from build123d import *

# Parameters (mm, degrees)
SZKIC1_R                    = 15
DODANIE_WYCI_GNI_CIE1_DEPTH = 33
SZKIC2_R                    = 20
DODANIE_WYCI_GNI_CIE2_DEPTH = 2
SZKIC3_R                    = 44
DODANIE_WYCI_GNI_CIE3_DEPTH = 15
SZKIC4_R                    = 15
DODANIE_WYCI_GNI_CIE4_DEPTH = 10


with BuildPart() as part:
    # Szkic1 → Dodanie-wyciągnięcie1 (new body)
    with BuildSketch(Plane.XY):
        Circle(SZKIC1_R)
    extrude(amount=DODANIE_WYCI_GNI_CIE1_DEPTH)

    # Szkic2 → Dodanie-wyciągnięcie2 (add)
    with BuildSketch(Plane(origin=(0, 0, 0), x_dir=(-1, 0, 0), z_dir=(0, 0, -1))):
        Circle(SZKIC2_R)
    extrude(amount=DODANIE_WYCI_GNI_CIE2_DEPTH)

    # Szkic3 → Dodanie-wyciągnięcie3 (add)
    with BuildSketch(Plane(origin=(0, 0, -2), x_dir=(-1, 0, 0), z_dir=(0, 0, -1))):
        Circle(SZKIC3_R)
    extrude(amount=DODANIE_WYCI_GNI_CIE3_DEPTH)

    # Szkic4 → Dodanie-wyciągnięcie4 (add)
    with BuildSketch(Plane(origin=(0, 0, -17), x_dir=(-1, 0, 0), z_dir=(0, 0, -1))):
        with Locations((0, 20)):
            Circle(SZKIC4_R)
    extrude(amount=DODANIE_WYCI_GNI_CIE4_DEPTH)

    # Lustro1: part across plane


with BuildPart() as part_1:
    add(part.part)
    add(part.part.mirror(Plane(origin=(0, 20, -27), x_dir=(1, 0, 0), z_dir=(0, 0, -1))))


solid = part_1.part
Design review of the part built by this model. Coordinates are the model's own, in mm. A direction names the side the tool comes from. Round coordinates to 2 decimals unless told otherwise and drop trailing zeros. Order: outer loops, then holes, each group sorted by start corner. A loop starts at its lowest first (then second) coordinate and runs counter-clockwise, first axis right, second up. Notation, with made-up numbers: M 43.5,2.5 L 88.5,2.5 A24 cw 88.5,21.5 Z; hole C 27.25,85.5 d11. An arc over 180 degrees is marked long. Answer as CSV lines item,"result". Start each with the question number.
1) The part is to be moulded in two halves that separate along Z. For faces 4 (the face through (-3, 15, -54)), 5 (the face through (-14.985, 0.66, -70.269)), 6 (the face through (1, 1, -37)), say which applies: +Z half, -Z half, draft (parallel to the pull), parting line (faces both ways), or undercut.
2) Add section D-D (z = -75). Give the boundary of the cut face in (x, y).
3) Add section A-A (x = 0). Give the boundary of the cut face in (y, z).
4) Add section C-C (x = 39). Give the boundary of the cut face in (y, z), then the cut area to 3 significant figures.
5) For pin 1 Ø10 at (x, z) = (22.5, 11) entering from -Y; pin 2 Ø5 at (x, z) = (-27, -18.5) entering from +Y; pin 3 Ø1.5 at (x, y) = (-23.5, 30) entering from -Z; pin 4 Ø1 at (y, z) = (-31.5, -10.5) entering from +X (3 decimals), all flat-tipped, find the tip position at first contact; note any pin that passes through.
6) Wall thickness on line 1 along Z through (x, y) = (19, 19); line 2 along Z through (x, y) = (18, 0); line 3 along Y through (x, z) = (1, -38): over which ranges is each line inside the solid? List them lowest first. Write a range as [from, to].
7) Tool access review of faces 1 (the face through (9.538, -42.954, -9.395)), 2 (the face through (4.336, -19.524, -53.014)), 3 (the face through (-9, -19, -2)): name each direction out of +Z, -Z, +X, -X, +Y, -Y from which nothing blocks a thin tool from reaching the whole face with its end or side.
8) Add section B-B (y = 0). Give the boundary of the cut face in (x, z), then the cut area to 3 significant figures.
Resolved:
1,face 4,"-Z half"
1,face 5,"draft"
1,face 6,"undercut"
2,outline,"C 0,0 d30"
3,outline,"M -44,-52 L -20,-52 L -20,-54 L -15,-54 L -15,-87 L 15,-87 L 15,-54 L 20,-54 L 20,-52 L 44,-52 L 44,-37 L 35,-37 L 35,-17 L 44,-17 L 44,-2 L 20,-2 L 20,0 L 15,0 L 15,33 L -15,33 L -15,0 L -20,0 L -20,-2 L -44,-2 L -44,-17 L 5,-17 L 5,-37 L -44,-37 Z"
4,outline,"M -20.37,-52 L 20.37,-52 L 20.37,-37 L -20.37,-37 Z; M -20.37,-17 L 20.37,-17 L 20.37,-2 L -20.37,-2 Z"
4,area,"1,220 mm^2"
5,pin 1,"through"
5,pin 2,"y = 36.21"
5,pin 3,"z = -52"
5,pin 4,"x = 31.225"
6,line 1,"[-52, -37], [-17, -2]"
6,line 2,"[-54, -37], [-17, 0]"
6,line 3,"[-43.99, 43.99]"
7,face 1,"+Z, -Z"
7,face 2,"-Z"
7,face 3,"+Z"
8,outline,"M -44,-52 L -20,-52 L -20,-54 L -15,-54 L -15,-87 L 15,-87 L 15,-54 L 20,-54 L 20,-52 L 44,-52 L 44,-37 L -44,-37 Z; M -44,-17 L 44,-17 L 44,-2 L 20,-2 L 20,0 L 15,0 L 15,33 L -15,33 L -15,0 L -20,0 L -20,-2 L -44,-2 Z"
8,area,"4,780 mm^2"
